Check sheet for the modelled part. Datum: model origin and axes. Units: mm. A direction names the side the tool comes from. Give positions to 0.01 mm unless a question says otherwise; leave off trailing zeros. Loops run counter-clockwise (first coordinate to the right, second up) from the corner with the lowest first, then second, coordinate; pieces in that order, holes last. Notation, with made-up numbers: M 74.25,-7 L 98.25,-7 A33 cw 98.25,26 Z; hole C 10.5,30.25 d8. An arc over 180 degrees is marked long. Write each question's results on one line, items separated by ' | '. Start each with the question number.
1. Draft check along X on faces 5 (the flat face through (0, 0, 0)), 6 (the cylindrical face through (-69, 3.2, -0.52)), 7 (the flat face through (-64, -1, -6.668)). Enter one of: pulls with the +X half, pulls with the -X half, needs draft (parallel to the pull), parting line crosses it, or undercut.
2. Material ranges on line 1 along X through (y, z) = (1.5, 0) (3 decimals); line 2 along X through (y, z) = (1, 14); line 3 along Y through (x, z) = (-56, 0.5) (1 decimal), recorded low to high.
3. Tool access check on faces 1 (the flat face through (-13, -3, 6.35)), 2 (the flat face through (-73.025, 2, 0)), 3 (the flat face through (-61, 0, -12.7)), 4 (the flat face through (-62, -3.175, 3)). Record the directions out of +Z, -Z, +X, -X, +Y, -Y that give a thin tool (end or side, any length) a straight path to the whole face; none if there is none.
4. Sectioned sample at D-D on y = 0.25. Give the number of separate pieces and of enclosed holes in the cut face, and give its area (3 significant figures).
5. Sectioned sample at B-B on z = 0. Record the cut outline in (x, y) (1 decimal), and give its area (3 significant figures).
6. Sectioned sample at C-C on x = -59. Record the cut outline in (y, z) (1 decimal).
7. Sectioned sample at A-A on x = -24.13. Record the cut outline in (y, z) (1 decimal), and give its area (3 significant figures).
8. Go/stop test with flat-tipped pins: pin 1 (2 mm diameter, centred on y = 1, z = 10.5, fed in from -X); pin 2 (1 mm diameter, centred on x = -12, y = -2.5, fed in from +Z); pin 3 (1 mm diameter, centred on y = 0, z = 11, fed in from -X). Record where each tip stops, or that it passes through.
```python
from build123d import *

# Parameters (mm, degrees)
SKETCH1_W           = 50.8
SKETCH1_H           = 9.525
BOSS_EXTRUDE1_DEPTH = 73.025
CUT_EXTRUDE2_DEPTH  = 19.05
SKETCH4_R           = 2.38125
CUT_EXTRUDE3_DEPTH  = 78.90081033
SKETCH5_W           = 12.7
SKETCH5_H           = 9.525
CUT_EXTRUDE4_DEPTH  = 29.21
FILLET2_R           = 8.89
FILLET3_R           = 3.81
FILLET4_R           = 13.97
FILLET5_R           = 13.97
CUT_EXTRUDE10_DEPTH = 3.175
SKETCH14_R          = 3.175
CUT_EXTRUDE11_DEPTH = 78.576627575
SKETCH17_R          = 2.38125
CUT_EXTRUDE12_DEPTH = 78.900810468
SKETCH19_W          = 19.05
SKETCH19_H          = 4.7625
CUT_EXTRUDE14_DEPTH = 6.0325
FILLET8_R           = 3.81
FILLET9_R           = 3.81


with BuildPart() as part:
    # Sketch1 → Boss-Extrude1 (new body)
    with BuildSketch(Plane(origin=(0, 0, 0), x_dir=(0, 0, -1), z_dir=(1, 0, 0))):
        Rectangle(SKETCH1_W, SKETCH1_H)
    extrude(amount=-BOSS_EXTRUDE1_DEPTH)

    # Sketch3 → Cut-Extrude2 (cut)
    with BuildSketch(Plane.ZY.offset(73.025)):
        Polygon((-6.6675, -3.175), (6.6675, -3.175), (6.6675, -0.79375), (6.6675, 1.5875), (-6.6675, 1.5875), (-6.6675, -0.79375), align=None)
    extrude(amount=-CUT_EXTRUDE2_DEPTH, mode=Mode.SUBTRACT)

    # Sketch4 → Cut-Extrude3 (cut, through all)
    with BuildSketch(Plane(origin=(0, 4.7625, 0), x_dir=(1, 0, 0), z_dir=(0, 1, 0))):
        with Locations(Location((-66.675, 0, 0), (0, 0, 270))):
            Circle(SKETCH4_R)
    extrude(amount=-CUT_EXTRUDE3_DEPTH, mode=Mode.SUBTRACT)

    # Sketch5 → Cut-Extrude4 (cut)
    with BuildSketch(Plane.ZY.offset(73.025)):
        with Locations((-19.05, 0)):
            Rectangle(SKETCH5_W, SKETCH5_H)
        with Locations((19.05, 0)):
            Rectangle(SKETCH5_W, SKETCH5_H)
    extrude(amount=-CUT_EXTRUDE4_DEPTH, mode=Mode.SUBTRACT)

    # Fillet2
    fillet2_edges = [part.edges().sort_by_distance(p)[0] for p in [
        (-43.815, 0, -12.7),
        (-43.815, 0, 12.7),
    ]]
    fillet(fillet2_edges, radius=FILLET2_R)

    # Fillet3
    fillet3_edges = [part.edges().sort_by_distance(p)[0] for p in [
        (-73.025, 0, -12.7),
    ]]
    fillet(fillet3_edges, radius=FILLET3_R)

    # Fillet4
    fillet4_edges = [part.edges().sort_by_distance(p)[0] for p in [
        (-43.815, 0, 25.4),
        (-43.815, 0, -25.4),
    ]]
    fillet(fillet4_edges, radius=FILLET4_R)

    # Fillet5
    fillet5_edges = [part.edges().sort_by_distance(p)[0] for p in [
        (0, 0, 25.4),
        (0, 0, -25.4),
    ]]
    fillet(fillet5_edges, radius=FILLET5_R)

    # Sketch13 → Cut-Extrude10 (cut)
    with BuildSketch(Plane.XZ.offset(4.7625)):
        with BuildLine():
            Line((-30.48, 6.35), (-30.48, 15.08125))
            ThreePointArc((-30.48, 15.08125), (-24.13, 21.43125), (-17.78, 15.08125))
            Line((-17.78, 15.08125), (-17.78, 6.35))
            Line((-17.78, 6.35), (-8.255, 6.35))
            ThreePointArc((-8.255, 6.35), (-1.905, 0), (-8.255, -6.35))
            Line((-8.255, -6.35), (-17.78, -6.35))
            Line((-17.78, -6.35), (-17.78, -15.08125))
            ThreePointArc((-17.78, -15.08125), (-24.13, -21.43125), (-30.48, -15.08125))
            Line((-30.48, -15.08125), (-30.48, -6.35))
            Line((-30.48, -6.35), (-40.005, -6.35))
            ThreePointArc((-40.005, -6.35), (-46.355, 0), (-40.005, 6.35))
            Line((-40.005, 6.35), (-30.48, 6.35))
        make_face()
    extrude(amount=-CUT_EXTRUDE10_DEPTH, mode=Mode.SUBTRACT)

    # Sketch14 → Cut-Extrude11 (cut, through all)
    with BuildSketch(Plane.XZ.offset(1.5875)):
        with Locations(Location((-24.13, 0, 0), (0, 0, 270))):
            Circle(SKETCH14_R)
    extrude(amount=-CUT_EXTRUDE11_DEPTH, mode=Mode.SUBTRACT)

    # Sketch17 → Cut-Extrude12 (cut, through all)
    with BuildSketch(Plane(origin=(0, -4.7625, 0), x_dir=(-1, 0, 0), z_dir=(0, -1, 0))):
        with Locations(Location((40.005, -12.7, 0), (0, 0, 90))):
            Circle(SKETCH17_R)
        with Locations(Location((40.005, 12.7, 0), (0, 0, 90))):
            Circle(SKETCH17_R)
        with Locations(Location((8.255, -12.7, 0), (0, 0, 90))):
            Circle(SKETCH17_R)
        with Locations(Location((8.255, 12.7, 0), (0, 0, 90))):
            Circle(SKETCH17_R)
    extrude(amount=-CUT_EXTRUDE12_DEPTH, mode=Mode.SUBTRACT)

    # Sketch19 → Cut-Extrude14 (cut)
    with BuildSketch(Plane.XY.offset(12.7)):
        with Locations((-63.5, -0.79375)):
            Rectangle(SKETCH19_W, SKETCH19_H)
    extrude(amount=-CUT_EXTRUDE14_DEPTH, mode=Mode.SUBTRACT)

    # Fillet8
    # the kernel refuses this fillet: 3.81 mm, written as the material it takes off along each edge
    with BuildSketch(Plane(origin=(-53.975, 1.5875, 12.7), x_dir=(0, 0, -1), z_dir=(0, -1, 0))) as fillet8_piece_1:
        with BuildLine():
            CenterArc((3.553407893, 3.81), FILLET8_R, 191.536959033, 78.463040967)
            Line((-0.179614475, 3.048), (-0.552916711, 2.9718))
            ThreePointArc((-0.552916711, 2.9718), (-0.381, 1.27), (-0.381, 0))
            Line((-0.381, 0), (0, -0.381))
            Line((0, -0.381), (3.553407893, -0.381))
            Line((3.553407893, -0.381), (3.553407893, 0))
        make_face()
    extrude(amount=4.7625, mode=Mode.SUBTRACT)

    # Fillet9
    fillet9_edges = [part.edges().sort_by_distance(p)[0] for p in [
        (-73.025, -3.96875, 12.7),
        (-73.025, 3.175, 12.7),
    ]]
    fillet(fillet9_edges, radius=FILLET9_R)


solid = part.part
```
Output values:
1) face 5: pulls with the +X half | face 6: undercut | face 7: needs draft
2) line 1: -53.975 to -27.305, -20.955 to 0 | line 2: -48.08 to -42, -38.01 to -10.25, -6.26 to -0.24 | line 3: -4.8 to -3.2, 1.6 to 4.8
3) face 1: -Y | face 2: +Z, -Z, -X, +Y, -Y | face 3: -Z, -X, +Y, -Y | face 4: +Z, -X
4) separate pieces: 1 | enclosed holes: 5 | area: 2,400 mm2
5) outline: M -73,-4.8 L -69.1,-4.8 L -69.1,-3.2 L -73,-3.2 Z; M -73,1.6 L -69.1,1.6 L -69.1,4.8 L -73,4.8 Z; M -64.3,-4.8 L -46.4,-4.8 L -46.4,-1.6 L -27.3,-1.6 L -27.3,4.8 L -64.3,4.8 L -64.3,1.6 L -54,1.6 L -54,-3.2 L -64.3,-3.2 Z; M -21,-1.6 L -1.9,-1.6 L -1.9,-4.8 L 0,-4.8 L 0,4.8 L -21,4.8 Z | area: 401 mm2
6) outline: M -4.8,-12.7 L 4.8,-12.7 L 4.8,12.7 L 1.6,12.7 L 1.6,-6.7 L -3.2,-6.7 L -3.2,12.7 L -4.8,12.7 Z
7) outline: M -4.8,-25.4 L 4.8,-25.4 L 4.8,-3.2 L -1.6,-3.2 L -1.6,-21.4 L -4.8,-21.4 Z; M -4.8,21.4 L -1.6,21.4 L -1.6,3.2 L 4.8,3.2 L 4.8,25.4 L -4.8,25.4 Z | area: 307 mm2
8) pin 1: x = -72.94 | pin 2: z = 25.32 | pin 3: x = -53.73
